Verification items for the finished model (mm, model axes). Face numbers are marked on the shaded views. Coordinates: 2 decimals unless noted, no trailing zeros. Write each loop counter-clockwise with the first axis right and the second up, starting at its lowest first coordinate (ties: lowest second). Pieces come first, ordered by that corner, then holes. Notation, with made-up numbers: (20, -0.5) -> (45, -0.5) arc R21 cw to (45, 31.5) -> close; hole circle Ø4 at (64, -33.75). An arc over 180 degrees is marked (long way). Write each question's results on one line, items separated by ' | '. Start each with the question number.
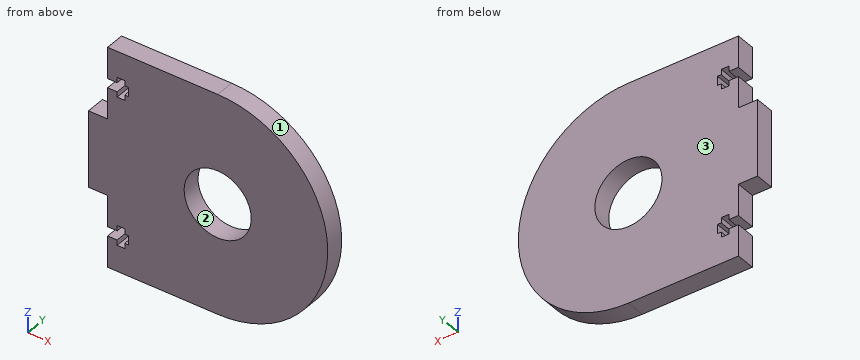
from build123d import *

# Parameters (mm, degrees)
SKETCH1_R           = 11.1379
BOSS_EXTRUDE1_DEPTH = 6.35


with BuildPart() as part:
    # Sketch1 → Boss-Extrude1 (new body)
    with BuildSketch(Plane(origin=(0, 0, 0), x_dir=(1, 0, 0), z_dir=(0, 1, 0))):
        with BuildLine():
            Line((-34.169803213, 12.296548394), (-40.519803213, 12.296548394))
            Line((-40.519803213, 12.296548394), (-40.519803213, -13.103451606))
            Line((-40.519803213, -13.103451606), (-34.169803213, -13.103451606))
            Line((-34.169803213, -13.103451606), (-34.169803213, -23.498436767))
            Line((-34.169803213, -23.498436767), (-30.994803213, -23.498436767))
            Line((-30.994803213, -23.498436767), (-30.994803213, -21.745836767))
            Line((-30.994803213, -21.745836767), (-28.454803213, -21.745836767))
            Line((-28.454803213, -21.745836767), (-28.454803213, -23.498436767))
            Line((-28.454803213, -23.498436767), (-27.184803213, -23.498436767))
            Line((-27.184803213, -23.498436767), (-27.184803213, -26.546296123))
            Line((-27.184803213, -26.546296123), (-28.454803213, -26.546296123))
            Line((-28.454803213, -26.546296123), (-28.454803213, -28.298896123))
            Line((-28.454803213, -28.298896123), (-30.994803213, -28.298896123))
            Line((-30.994803213, -28.298896123), (-30.994803213, -26.546296123))
            Line((-30.994803213, -26.546296123), (-34.169803213, -26.546296123))
            Line((-34.169803213, -26.546296123), (-34.169803213, -36.941351606))
            Line((-34.169803213, -36.941351606), (2.368096787, -36.941351606))
            ThreePointArc((2.368096787, -36.941351606), (38.905996787, -0.403451606), (2.368096787, 36.134448394))
            Line((2.368096787, 36.134448394), (-34.169803213, 36.134448394))
            Line((-34.169803213, 36.134448394), (-34.169803213, 25.739463233))
            Line((-34.169803213, 25.739463233), (-30.994803213, 25.739463233))
            Line((-30.994803213, 25.739463233), (-30.994803213, 27.492063233))
            Line((-30.994803213, 27.492063233), (-28.454803213, 27.492063233))
            Line((-28.454803213, 27.492063233), (-28.454803213, 25.739463233))
            Line((-28.454803213, 25.739463233), (-27.184803213, 25.739463233))
            Line((-27.184803213, 25.739463233), (-27.184803213, 22.691603877))
            Line((-27.184803213, 22.691603877), (-28.454803213, 22.691603877))
            Line((-28.454803213, 22.691603877), (-28.454803213, 20.939003877))
            Line((-28.454803213, 20.939003877), (-30.994803213, 20.939003877))
            Line((-30.994803213, 20.939003877), (-30.994803213, 22.691603877))
            Line((-30.994803213, 22.691603877), (-34.169803213, 22.691603877))
            Line((-34.169803213, 22.691603877), (-34.169803213, 12.296548394))
        make_face()
        with Locations(Location((2.368096787, -0.403451606, 0), (0, 0, 270))):
            Circle(SKETCH1_R, mode=Mode.SUBTRACT)
    extrude(amount=BOSS_EXTRUDE1_DEPTH)


solid = part.part
1. Sectioned sample at D-D on z = 32.5. Record the cut outline in (x, y).
2. Depth check by flat-ended pin: pin 1 Ø1.9 at (y, z) = (2, 22.5) entering from -X; pin 2 Ø1.5 at (x, z) = (-2, 21) entering from -Y; pin 3 Ø1.9 at (x, y) = (-39, 2) entering from +Z; pin 4 Ø2.5 at (y, z) = (4, 25) entering from -X. Enter the tip coordinate at first touch or a pass-through.
3. Mould release check, pull along X, two halves, no side actions. Record for the marked faces 1, 2 and 3: +X half, -X half, draft (parallel to the pull), parting line (faces both ways), or undercut.
4. Material ranges on probe 1 along Z at (x, y) = (-28, 1.5); probe 2 along X at (y, z) = (1.5, 6); probe 3 along X at (y, z) = (0.75, 5), recorded low to high. Write a range as from..to.
5. Sectioned sample at C-C on x = 9.5. Record the cut outline in (y, z).
6. Sectioned sample at B-B on z = -4. Record the cut outline in (x, y), plus the area to 3 significant figures.
Computed values:
1) outline: (-34.17, 0) -> (19.83, 0) -> (19.83, 6.35) -> (-34.17, 6.35) -> close
2) pin 1: stops at x = -34.17 | pin 2: stops at y = 0 | pin 3: stops at z = 13.1 | pin 4: stops at x = -27.18
3) face 1: +X half | face 2: undercut | face 3: draft
4) probe 1: z = -36.13..-25.74, -22.69..23.5, 26.55..36.94 | probe 2: x = -40.52..-7.26, 12..38.47 | probe 3: x = -40.52..-7.78, 12.51..38.62
5) outline: (0, -35.43) -> (6.35, -35.43) -> (6.35, -8.15) -> (0, -8.15) -> close; (0, 8.96) -> (6.35, 8.96) -> (6.35, 36.24) -> (0, 36.24) -> close
6) outline: (-40.52, 0) -> (-7.86, 0) -> (-7.86, 6.35) -> (-40.52, 6.35) -> close; (12.6, 0) -> (38.64, 0) -> (38.64, 6.35) -> (12.6, 6.35) -> close | area: 373 mm^2
